Model file for the job. Use its own axes, mm. Face numbers are marked on the shaded views. A direction names the side the tool comes from. Give positions to 0.01 mm unless a question says otherwise; leave off trailing zeros. Order: outer loops, then holes, each group sorted by start corner. A loop starts at its lowest first (then second) coordinate and runs counter-clockwise, first axis right, second up. Notation, with made-up numbers: (-8, -25) - (9, -25) arc R16 cw to (9, -19) - close; hole circle Ø10 at (-33, 34). An arc over 180 degrees is marked (long way). Use CSV: the item, a comma, the result in double quotes. Start each with the question number.
(1) Probe L1, parallel to Y at x = 1.75, z = -13.5; L2, parallel to Y at x = 4.5, z = -9; L3, parallel to Z at x = 4, y = -2.5. List the from-to ranges inside material, lowest first.
(2) Tool access for the marked faces 4 and 5: list every direction of +Z, -Z, +X, -X, +Y, -Y with a clear straight run to the whole face (end or side of a thin tool).
(3) Pull direction Z, two halves, no side cores. Call the marked faces 1, 2 and 3: +Z half, -Z half, draft (parallel to the pull), parting line (faces both ways), or undercut.
(4) Band-saw the part on A-A, the plane z = 0. Give the cut face in (x, y), then the cut area to 3 significant figures.
(5) Drop flat-ended pins along their axis: pin 1 Ø3 at (x, z) = (3, 11) entering from +Y; pin 2 Ø2 at (x, y) = (8.5, -34.5) entering from +Z; pin 3 Ø5 at (x, z) = (6.5, 25.5) entering from -Y. Give the stop position or say it passes through.
(6) Band-saw the part on D-D, the plane y = 40.5. Give the cut face in (x, z), then the cut area to 3 significant figures.
(7) Band-saw the part on B-B, the plane x = 3. Count the separate pieces of the cut face and the enclosed holes in it, then the cut area to 3 significant figures.
Autodesk Inventor part; units mm, degrees
ref_plane "YZ Plane" through (0, 0, 0) normal (1, 0, 0) x (0, 1, 0)
ref_plane "XZ Plane" through (0, 0, 0) normal (0, 1, 0) x (-1, 0, 0)
ref_plane "XY Plane" through (0, 0, 0) normal (0, 0, 1) x (1, 0, 0)
sketch "Sketch2" plane through (0, 0, 0) normal (1, 0, 0) x (0, 1, 0)
  circle A0 centre (0, 0) radius 54.5
  circle A1 centre (-27.25, -35.3988) radius 3.5
  circle A2 centre (-27.25, 35.3988) radius 3.5
  circle A3 centre (27.25, -35.3988) radius 3.5
  circle A4 centre (27.25, 35.3988) radius 3.5
  circle A5 centre (0, 0) radius 21.5
extrude "Extrusion4" add sketch "Sketch2" along normal blind 10
sketch "Sketch4" plane through (10, 0, 0) normal (1, 0, 0) x (0, 0, -1)
  circle A0 centre (0, 0) radius 54.5
  circle A1 centre (0, 0) radius 21.5
  arc A2 (10, 38) -> (-10, 38) centre (0, 26.8197) ccw construction
  arc A3 (13.4228, 41.8269) -> (-13.4228, 41.8269) centre (0, 26.8197) ccw
  arc A4 (6.5772, 34.1731) -> (-6.5772, 34.1731) centre (0, 26.8197) ccw
  arc A5 (6.5772, 34.1731) -> (13.4228, 41.8269) centre (10, 38) ccw
  arc A6 (-13.4228, 41.8269) -> (-6.5772, 34.1731) centre (-10, 38) ccw
  dimension "d28" = 15
extrude "Extrusion5" cut sketch "Sketch4" against normal blind 10 contours A5 A4 A6 A3
pattern_circular "Circular Pattern2" count 4 over 360 about axis through (0, 0, 0) along (1, 0, 0) of "Extrusion5"
sketch "Sketch5" plane through (10, 0, 0) normal (1, 0, 0) x (0, 0, -1)
  arc A0 (41.8269, 13.4228) -> (34.1731, 6.5772) centre (38, 10) ccw
  arc A1 (41.8269, -13.4228) -> (41.8269, 13.4228) centre (26.8197, 0) ccw
  arc A2 (34.1731, -6.5772) -> (41.8269, -13.4228) centre (38, -10) ccw
  arc A3 (34.1731, -6.5772) -> (34.1731, 6.5772) centre (26.8197, 0) ccw
  arc A4 (13.4228, -41.8269) -> (6.5772, -34.1731) centre (10, -38) ccw
  arc A5 (-13.4228, -41.8269) -> (13.4228, -41.8269) centre (0, -26.8197) ccw
  arc A6 (-6.5772, -34.1731) -> (-13.4228, -41.8269) centre (-10, -38) ccw
  arc A7 (-6.5772, -34.1731) -> (6.5772, -34.1731) centre (0, -26.8197) ccw
  arc A8 (-41.8269, -13.4228) -> (-34.1731, -6.5772) centre (-38, -10) ccw
  arc A9 (-41.8269, 13.4228) -> (-41.8269, -13.4228) centre (-26.8197, 0) ccw
  arc A10 (-34.1731, 6.5772) -> (-41.8269, 13.4228) centre (-38, 10) ccw
  arc A11 (-34.1731, 6.5772) -> (-34.1731, -6.5772) centre (-26.8197, 0) ccw
  arc A12 (-13.4228, 41.8269) -> (-6.5772, 34.1731) centre (-10, 38) ccw
  arc A13 (13.4228, 41.8269) -> (-13.4228, 41.8269) centre (0, 26.8197) ccw
  arc A14 (6.5772, 34.1731) -> (13.4228, 41.8269) centre (10, 38) ccw
  arc A15 (6.5772, 34.1731) -> (-6.5772, 34.1731) centre (0, 26.8197) ccw
  circle A16 centre (0, 0) radius 21.5
  circle A17 centre (35.3988, 27.25) radius 3.5
  circle A18 centre (-35.3988, 27.25) radius 3.5
  circle A19 centre (-35.3988, -27.25) radius 3.5
  circle A20 centre (35.3988, -27.25) radius 3.5
  circle A21 centre (0, 0) radius 54.5
sketch "Sketch6" plane through (10, 0, 0) normal (1, 0, 0) x (0, 0, -1)
  circle A0 centre (-35.3988, 27.25) radius 3.5
  circle A1 centre (35.3988, 27.25) radius 3.5
  circle A2 centre (-35.3988, -27.25) radius 3.5
  circle A3 centre (35.3988, -27.25) radius 3.5
  circle A4 centre (-35.3988, 27.25) radius 4
  circle A5 centre (35.3988, 27.25) radius 4
  circle A6 centre (-35.3988, -27.25) radius 4
  circle A7 centre (35.3988, -27.25) radius 4
  point P0 (0, 0)
extrude "Extrusion6" cut sketch "Sketch6" against normal blind 10
properties part number "ballast_tutup"
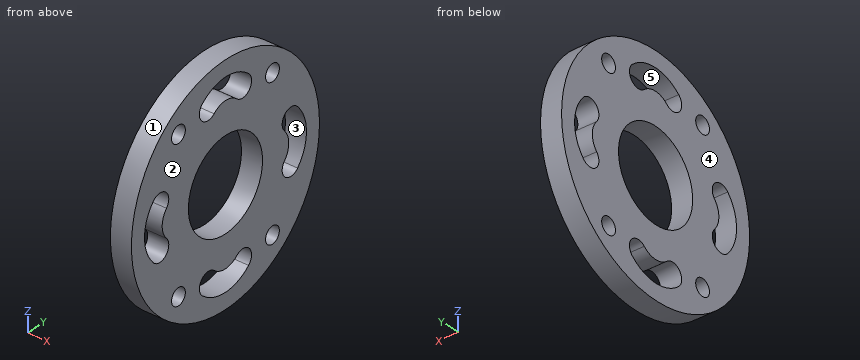
Answer block:
1,L1,"y = -52.8 to -41.76, -34.24 to -16.73, 16.73 to 34.24, 41.76 to 52.8"
1,L2,"y = -53.75 to -44.83, -32.96 to -19.53, 19.53 to 32.96, 44.83 to 53.75"
1,L3,"z = -54.44 to -46.8, -36.36 to -21.35, 21.35 to 36.36, 46.8 to 54.44"
2,face 4,"+Z, -Z, -X, +Y, -Y"
2,face 5,"+X, -X"
3,face 1,"parting line"
3,face 2,"draft"
3,face 3,"undercut"
4,outline,"(0, -54.5) - (10, -54.5) - (10, -46.95) - (0, -46.95) - close; (0, -36.69) - (10, -36.69) - (10, -21.5) - (0, -21.5) - close; (0, 21.5) - (10, 21.5) - (10, 36.69) - (0, 36.69) - close; (0, 46.95) - (10, 46.95) - (10, 54.5) - (0, 54.5) - close"
4,area,"455 mm2"
5,pin 1,"stops at y = 53.67"
5,pin 2,"stops at z = 42.99"
5,pin 3,"stops at y = -49.41"
6,outline,"(0, -36.47) - (10, -36.47) - (10, -14.48) - (0, -14.48) - close; (0, 14.48) - (10, 14.48) - (10, 36.47) - (0, 36.47) - close"
6,area,"440 mm2"
7,separate pieces,"1"
7,enclosed holes,"9"
7,area,"6,450 mm2"
